The model under review builds one solid part; all positions refer to its coordinate system, in mm. A direction names the side the tool comes from. Coordinates: 2 decimals unless noted, no trailing zeros. Write each loop counter-clockwise with the first axis right and the second up, starting at its lowest first coordinate (ties: lowest second). Pieces come first, ordered by that corner, then holes. Notation, with made-up numbers: (-19.75, 2) - (31.25, 2) arc R4 ccw to (31.25, 8) - close; hole circle Ø5 at (38.5, 39.5). An arc over 180 degrees is marked (long way). Put each result on its own line as item: value. Start each with the question number.
Item 1: Consider section A-A on y = 5. Give the boundary of the cut face in (x, z) (3 decimals), then the cut area to 3 significant figures.
Item 2: For pin 1 (1.6 mm diameter, centred on x = -14, z = 1.5, fed in from +Y); pin 2 (8 mm diameter, centred on x = 4, y = 6, fed in from +Z); pin 3 (0.9 mm diameter, centred on y = 4, z = 1, fed in from -X) (3 decimals); pin 4 (0.9 mm diameter, centred on y = -4, z = 1, fed in from +X) (3 decimals), all flat-tipped, find the tip position at first contact; note any pin that passes through.
Item 3: Consider section C-C on x = 15. Give the boundary of the cut face in (y, z).
Item 4: Mouldability with a two-part tool opening along X and no side actions: class faces 1 (the face through (-1.575, 5, 2)), 2 (the face through (-7.775, 5, 2)), 3 (the face through (7.775, 5, 2)) as pulls with the +X half, pulls with the -X half, needs draft (parallel to the pull), parting line crosses it, or undercut.
Item 5: Machinability: for faces 4 (the face through (-17, 1.55, 2)), 5 (the face through (-1.575, -5, 2)), 6 (the face through (7.775, -5, 2)), 7 (the face through (-4.625, 5, 2)), 8 (the face through (-7.775, -5, 2)), which of the approach directions +Z, -Z, +X, -X, +Y, -Y give a long, thin tool a straight path to every point of the face, cutting with its end or side? Answer none if there is none.
Item 6: To check wall thickness, follow L1, parallel to X at y = 3.5, z = 1.65 (3 decimals); L2, parallel to Y at x = 22, z = 2.6. State the ranges of each line that lie inside material, in increasing order. Write a range as [from, to].
Item 7: Consider section B-B on z = 2.3. Give the boundary of the cut face in (x, y) (3 decimals).
Autodesk Inventor part; units mm, degrees
ref_plane "YZ Plane" through (0, 0, 0) normal (1, 0, 0) x (0, 1, 0)
ref_plane "XZ Plane" through (0, 0, 0) normal (0, 1, 0) x (-1, 0, 0)
ref_plane "XY Plane" through (0, 0, 0) normal (0, 0, 1) x (1, 0, 0)
sketch "tabs" plane through (0, 0, 0) normal (0, 0, 1) x (1, 0, 0)
  line L0 (15.6175, 17.0118) -> (18.7675, 17.0118)
  line L1 (18.7675, 17.0118) -> (18.7675, 10.7868)
  line L2 (18.7675, 10.7868) -> (15.6175, 10.7868)
  line L3 (15.6175, 10.7868) -> (15.6175, 17.0118)
  line L4 (21.8175, 17.0118) -> (24.9675, 17.0118)
  line L5 (24.9675, 17.0118) -> (24.9675, 10.7868)
  line L6 (24.9675, 10.7868) -> (21.8175, 10.7868)
  line L7 (21.8175, 10.7868) -> (21.8175, 17.0118)
  line L8 (28.0175, 17.0118) -> (31.1675, 17.0118)
  line L9 (31.1675, 17.0118) -> (31.1675, 10.7868)
  line L10 (31.1675, 10.7868) -> (28.0175, 10.7868)
  line L11 (28.0175, 10.7868) -> (28.0175, 17.0118)
  line L12 (23.3925, 10.7868) -> (23.3925, 8.8536) construction
  point P0 (23.3925, 12.1901)
  dimension "d2" = 3.15
  dimension "d3" = 3.05
  dimension "d4" = 3.05
  dimension "d5" = 6.225
sketch "Sketch1" plane through (0, 0, 0) normal (0, 0, 1) x (1, 0, 0)
  line L0 (-25, 1.55) -> (25, 1.55)
  line L1 (25, 1.55) -> (25, -1.55)
  line L2 (25, -1.55) -> (-25, -1.55)
  line L3 (-25, -1.55) -> (-25, 1.55)
  line L4 (0, 16.9043) -> (0, -20.0235) construction
  line L5 (-32.3473, 0) -> (40.4078, 0) construction
  line L6 (-7.775, 7.775) -> (-4.625, 7.775)
  line L7 (-4.625, 7.775) -> (-4.625, 1.55)
  line L8 (-4.625, 1.55) -> (-7.775, 1.55)
  line L9 (-7.775, 1.55) -> (-7.775, 7.775)
  line L10 (-1.575, 7.775) -> (1.575, 7.775)
  line L11 (1.575, 7.775) -> (1.575, 1.55)
  line L12 (1.575, 1.55) -> (-1.575, 1.55)
  line L13 (-1.575, 1.55) -> (-1.575, 7.775)
  line L14 (4.625, 7.775) -> (7.775, 7.775)
  line L15 (7.775, 7.775) -> (7.775, 1.55)
  line L16 (7.775, 1.55) -> (4.625, 1.55)
  line L17 (4.625, 1.55) -> (4.625, 7.775)
  line L18 (0, 1.55) -> (0, -0.3832) construction
  line L19 (-7.775, -1.55) -> (-4.625, -1.55)
  line L20 (-4.625, -1.55) -> (-4.625, -7.775)
  line L21 (-4.625, -7.775) -> (-7.775, -7.775)
  line L22 (-7.775, -7.775) -> (-7.775, -1.55)
  line L23 (-1.575, -1.55) -> (1.575, -1.55)
  line L24 (1.575, -1.55) -> (1.575, -7.775)
  line L25 (1.575, -7.775) -> (-1.575, -7.775)
  line L26 (-1.575, -7.775) -> (-1.575, -1.55)
  line L27 (4.625, -1.55) -> (7.775, -1.55)
  line L28 (7.775, -1.55) -> (7.775, -7.775)
  line L29 (7.775, -7.775) -> (4.625, -7.775)
  line L30 (4.625, -7.775) -> (4.625, -1.55)
  line L31 (0, -7.775) -> (0, -9.7082) construction
  point P0 (0, 0)
  point P1 (25, 0)
  dimension "d0" = 50
  dimension "d1" = 3.1
extrude "Extrusion1" add sketch "Sketch1" along normal blind 3.1
equation "\"d2\" = mat + kerf"
equation "\"d3\" = mat - kerf"
equation "\"d4\" = mat - kerf"
equation "\"d5\" = 2 * mat + 0.5 * kerf"
equation "\"d1\" = mat"
equation "\"d6\" = mat"
properties part number "link1"
Report:
1. outline: (-7.775, 0) - (-4.625, 0) - (-4.625, 3.1) - (-7.775, 3.1) - close; (-1.575, 0) - (1.575, 0) - (1.575, 3.1) - (-1.575, 3.1) - close; (4.625, 0) - (7.775, 0) - (7.775, 3.1) - (4.625, 3.1) - close
1. area: 29.3 mm²
2. pin 1: y = 1.55
2. pin 2: z = 3.1
2. pin 3: x = -7.775
2. pin 4: x = 7.775
3. outline: (-1.55, 0) - (1.55, 0) - (1.55, 3.1) - (-1.55, 3.1) - close
4. face 1: undercut
4. face 2: pulls with the -X half
4. face 3: pulls with the +X half
5. face 4: +Z, -Z, -X, +Y
5. face 5: +Z, -Z, -Y
5. face 6: +Z, -Z, +X, -Y
5. face 7: +Z, -Z, +Y
5. face 8: +Z, -Z, -X, -Y
6. L1: [-7.775, -4.625], [-1.575, 1.575], [4.625, 7.775]
6. L2: [-1.55, 1.55]
7. outline: (-25, -1.55) - (-7.775, -1.55) - (-7.775, -7.775) - (-4.625, -7.775) - (-4.625, -1.55) - (-1.575, -1.55) - (-1.575, -7.775) - (1.575, -7.775) - (1.575, -1.55) - (4.625, -1.55) - (4.625, -7.775) - (7.775, -7.775) - (7.775, -1.55) - (25, -1.55) - (25, 1.55) - (7.775, 1.55) - (7.775, 7.775) - (4.625, 7.775) - (4.625, 1.55) - (1.575, 1.55) - (1.575, 7.775) - (-1.575, 7.775) - (-1.575, 1.55) - (-4.625, 1.55) - (-4.625, 7.775) - (-7.775, 7.775) - (-7.775, 1.55) - (-25, 1.55) - close
